```python
from build123d import *

# Parameters (mm, degrees)
PAD_DEPTH            = 70
SKETCH001_W          = 11.887794
SKETCH001_H          = 46.78
POCKET_DEPTH         = 70.001
POCKET001_DEPTH      = 30
SKETCH003_R          = 1.9
POCKET002_DEPTH      = 40.001
SKETCH004_W          = 17
SKETCH004_H          = 23.314381
POCKET003_DEPTH      = 40.001
SKETCH005_W          = 35
SKETCH005_H          = 57.974789
POCKET004_DEPTH      = 26
SKETCH006_W          = 45.255611
SKETCH006_H          = 30.428207
POCKET005_DEPTH      = 28
POCKET005_DEPTH_BACK = -100
SKETCH007_W          = 26.242121
SKETCH007_H          = 29.741062
POCKET006_DEPTH      = 45
SKETCH008_W          = 15.625622
SKETCH008_H          = 14.392597
SKETCH008_W_2        = 24.610352
SKETCH008_H_2        = 31.67345
POCKET007_DEPTH      = 45
SKETCH009_R          = 1.9
POCKET008_DEPTH      = 13
SKETCH010_R          = 1.6
POCKET009_DEPTH      = 5
SKETCH014_W          = 10
SKETCH014_H          = 15
PAD001_DEPTH         = 23
SKETCH015_W          = 11
SKETCH015_H          = 38.184422
SKETCH015_W_2        = 19.881198
SKETCH015_H_2        = 10
PAD002_DEPTH         = 8
SKETCH013_R          = 1.9
POCKET010_DEPTH      = 17
SKETCH011_R          = 1.9
POCKET011_DEPTH      = 15
PAD003_DEPTH         = 5
SKETCH017_R          = 3
POCKET012_DEPTH      = 2


with BuildPart() as part:
    # Sketch → Pad (new body)
    with BuildSketch(Plane.XY):
        Polygon((0, 0), (45, 0), (45, -50), (-28, -50), (-28, 0), align=None)
    extrude(amount=PAD_DEPTH)

    # Sketch001 (on Face7 of Pad) → Pocket (cut, through all)
    with BuildSketch(Plane.XY.offset(70)):
        with Locations((34.056103, -28.39)):
            Rectangle(SKETCH001_W, SKETCH001_H)
    extrude(amount=-POCKET_DEPTH, mode=Mode.SUBTRACT)

    # Sketch002 (on Face5 of Pocket) → Pocket001 (cut)
    with BuildSketch(Plane.XY.offset(70)):
        Polygon((30, -5), (30, -65.096024), (-40.783405, -65.096024), (-40.783405, 12.994774), (20, 12.994774), (20, -5), align=None)
    extrude(amount=-POCKET001_DEPTH, mode=Mode.SUBTRACT)

    # Sketch003 (on Face6 of Pocket001) → Pocket002 (cut, through all)
    with BuildSketch(Plane.XY.offset(40)):
        with Locations((-22, -40)):
            Circle(SKETCH003_R)
        with Locations((22, -40)):
            Circle(SKETCH003_R)
    extrude(amount=-POCKET002_DEPTH, mode=Mode.SUBTRACT)

    # Sketch004 (on Face6 of Pocket002) → Pocket003 (cut, through all)
    with BuildSketch(Plane.XY.offset(40)):
        with Locations((0, -43.65719)):
            Rectangle(SKETCH004_W, SKETCH004_H)
    extrude(amount=-POCKET003_DEPTH, mode=Mode.SUBTRACT)

    # Sketch005 (on Face13 of Pocket003) → Pocket004 (cut)
    with BuildSketch(Plane.XZ.offset(50)):
        with Locations((0, 7.512606)):
            Rectangle(SKETCH005_W, SKETCH005_H)
    extrude(amount=-POCKET004_DEPTH, mode=Mode.SUBTRACT)

    # Sketch006 (on Face11 of Pocket004) → Pocket005 (cut, two sides)
    with BuildSketch(Plane.XZ.offset(24)) as pocket005_sk:
        with Locations((-10.127806, 6.785896)):
            Rectangle(SKETCH006_W, SKETCH006_H)
    extrude(amount=-POCKET005_DEPTH, mode=Mode.SUBTRACT)
    extrude(pocket005_sk.sketch, amount=-POCKET005_DEPTH_BACK, mode=Mode.SUBTRACT)

    # Sketch007 (on Face12 of Pocket005) → Pocket006 (cut)
    with BuildSketch(Plane.XZ.offset(50)):
        with Locations((20.733142, 3.968048)):
            Rectangle(SKETCH007_W, SKETCH007_H)
    extrude(amount=-POCKET006_DEPTH, mode=Mode.SUBTRACT)

    # Sketch008 (on Face14 of Pocket006) → Pocket007 (cut)
    with BuildSketch(Plane.XZ.offset(50)):
        with Locations((42.909006, 69.196298)):
            Rectangle(SKETCH008_W, SKETCH008_H)
        with Locations((46.359665, 3.163275)):
            Rectangle(SKETCH008_W_2, SKETCH008_H_2)
    extrude(amount=-POCKET007_DEPTH, mode=Mode.SUBTRACT)

    # Sketch009 (on Face3 of Pocket007) → Pocket008 (cut)
    with BuildSketch(Plane.YZ.offset(45)):
        with Locations((-44, 55)):
            Circle(SKETCH009_R)
        with Locations((-13, 24)):
            Circle(SKETCH009_R)
        with Locations((-13, 55)):
            Circle(SKETCH009_R)
        with Locations((-44, 24)):
            Circle(SKETCH009_R)
    extrude(amount=-POCKET008_DEPTH, mode=Mode.SUBTRACT)

    # Sketch010 (on Face1 of Pocket008) → Pocket009 (cut)
    with BuildSketch(Plane(origin=(0, 0, 0), x_dir=(-1, 0, 0), z_dir=(0, 1, 0))):
        with Locations((-33, 5)):
            Circle(SKETCH010_R)
        with Locations((-40, 65)):
            Circle(SKETCH010_R)
        with Locations((-26, 65)):
            Circle(SKETCH010_R)
    extrude(amount=-POCKET009_DEPTH, mode=Mode.SUBTRACT)

    # Sketch014 (on Face4 of Pocket009) → Pad001 (join)
    with BuildSketch(Plane.YZ.offset(45)):
        with Locations((-30, 32.5)):
            Rectangle(SKETCH014_W, SKETCH014_H)
    extrude(amount=-PAD001_DEPTH)

    # Sketch015 (on Face29 of Pad001) → Pad002 (join)
    with BuildSketch(Plane(origin=(-28, 0, 0), x_dir=(0, -1, 0), z_dir=(-1, 0, 0))):
        with Locations((13.5, 54.907789)):
            Rectangle(SKETCH015_W, SKETCH015_H)
        with Locations((52.059401, 30)):
            Rectangle(SKETCH015_W_2, SKETCH015_H_2)
    extrude(amount=-PAD002_DEPTH)

    # Sketch013 (on Face19 of Pad002) → Pocket010 (cut)
    with BuildSketch(Plane.XZ.offset(24)):
        with Locations((-7, 27)):
            Circle(SKETCH013_R)
        with Locations((7, 27)):
            Circle(SKETCH013_R)
    extrude(amount=-POCKET010_DEPTH, mode=Mode.SUBTRACT)

    # Sketch011 (on Face29 of Pad002) → Pocket011 (cut)
    with BuildSketch(Plane(origin=(-28, 0, 0), x_dir=(0, -1, 0), z_dir=(-1, 0, 0))):
        with Locations((56.5, 30)):
            Circle(SKETCH011_R)
        with Locations((13, 68.5)):
            Circle(SKETCH011_R)
    extrude(amount=-POCKET011_DEPTH, mode=Mode.SUBTRACT)

    # Sketch016 (on Face1 of Pocket011) → Pad003 (join)
    with BuildSketch(Plane(origin=(0, 0, 0), x_dir=(-1, 0, 0), z_dir=(0, 1, 0))):
        Polygon((-12.5, 0), (5, 22), (-15.71, 22), align=None)
    extrude(amount=-PAD003_DEPTH)

    # Sketch017 (on Face28 of Pad003) → Pocket012 (cut)
    with BuildSketch(Plane.XZ.offset(5)):
        with Locations((26, 65)):
            Circle(SKETCH017_R)
        with Locations((33, 5)):
            Circle(SKETCH017_R)
        with Locations((40, 65)):
            Circle(SKETCH017_R)
    extrude(amount=-POCKET012_DEPTH, mode=Mode.SUBTRACT)


solid = part.part
```
The listing builds one solid part. Answer for the finished solid, in the listing's coordinates (mm). A direction names the side the tool comes from. Coordinates: 2 decimals unless noted, no trailing zeros. Write each loop counter-clockwise with the first axis right and the second up, starting at its lowest first coordinate (ties: lowest second). Pieces come first, ordered by that corner, then holes. Notation, with made-up numbers: (48, 75.25) - (65, 75.25) arc R22 ccw to (65, 98.25) - close; hole circle Ø9 at (86, -8.75). An arc over 180 degrees is marked (long way). Return JSON: item names as keys, results as strings. Group by question number.
1. A cutting plane is placed at C-C, the plane x = 22. Determine the outline of the cut face in (y, z), plus the area to 3 significant figures.
2. Determine the mould class of faces 4 (the flat face through (28.112, -23, 30)), 5 (the flat face through (29, -2, 0)), 6 (the flat face through (40, -28, 41)), 7 (the flat face through (12.5, -15, 20)) for opening direction X: released by +X, released by -X, zero draft, split by the parting line, or undercut.
3. A cutting plane is placed at D-D, the plane x = -22. Determine the outline of the cut face in (y, z), plus the area to 3 significant figures.
4. A cutting plane is placed at A-A, the plane y = -33.5. Determine the outline of the cut face in (x, z), plus the area to 3 significant figures.
5. A cutting plane is placed at B-B, the plane z = 65. Determine the outline of the cut face in (x, y), plus the area to 3 significant figures.
6. Which of the six approach directions +Z, -Z, +X, -X, +Y, -Y give full straight-line access (tool end or side, diameter ignored) to faces 1 (the flat face through (27.3, -3, 63.7)), 2 (the flat face through (0, -31, 36.5)), 3 (the cylindrical face through (42.535, -13.412, 53.145))?
7. Given pin 1 (2 mm diameter, centred on x = 31.5, y = -7.5, fed in from -Z); pin 2 (5 mm diameter, centred on x = 26, z = 65, fed in from -Y); pin 3 (10 mm diameter, centred on y = -45, z = 55, fed in from -X); pin 4 (2.5 mm diameter, centred on x = -23.5, z = 57.5, fed in from -Y), each flat-ended and moving along its own axis, determine where each tip first touches the part or whether it passes through.
8. Straight lines are drawn through the part: L1, parallel to X at y = -37, z = 27; L2, parallel to Z at x = 33, y = -0.8; L3, parallel to X at y = -17, z = 32.5. For each, find the intervals that lie inside material, in ascending order.
Ans:
{
 "1": {"outline": "(-50, 18.84) - (-41.9, 18.84) - (-41.9, 40) - (-50, 40) - close; (-38.1, 18.84) - (-5, 18.84) - (-5, 0) - (0, 0) - (0, 70) - (-5, 70) - (-5, 40) - (-38.1, 40) - close", "area": "1,220 mm²"},
 "2": {"face 4": "undercut", "face 5": "zero draft", "face 6": "undercut", "face 7": "released by -X"},
 "3": {"outline": "(-62, 25) - (-50, 25) - (-50, 22) - (-41.9, 22) - (-41.9, 40) - (-50, 40) - (-50, 35) - (-62, 35) - close; (-38.1, 22) - (0, 22) - (0, 40) - (-8, 40) - (-8, 74) - (-19, 74) - (-19, 40) - (-38.1, 40) - close; hole circle Ø3.8 at (-56.5, 30); hole circle Ø3.8 at (-13, 68.5)", "area": "1,300 mm²"},
 "4": {"outline": "(-28, 22) - (-17.5, 22) - (-17.5, 36.5) - (-8.5, 36.5) - (-8.5, 40) - (-28, 40) - close; (8.5, 36.5) - (17.5, 36.5) - (17.5, 18.84) - (28.11, 18.84) - (28.11, 25) - (40, 25) - (40, 19) - (45, 19) - (45, 62) - (40, 62) - (40, 40) - (8.5, 40) - close", "area": "870 mm²"},
 "5": {"outline": "(-28, -19) - (-20, -19) - (-20, -8) - (-28, -8) - close; (20, -5) - (23, -5) - (23, -3) - (24.4, -3) - (24.4, 0) - (20, 0) - close; (27.6, -3) - (29, -3) - (29, -5) - (37, -5) - (37, -3) - (38.4, -3) - (38.4, 0) - (27.6, 0) - close; (41.6, -3) - (43, -3) - (43, -5) - (45, -5) - (45, 0) - (41.6, 0) - close", "area": "170 mm²"},
 "6": {"face 1": "-Y", "face 2": "-Z, -Y", "face 3": "+X"},
 "7": {"pin 1": "through", "pin 2": "y = -3", "pin 3": "x = 40", "pin 4": "y = -19"},
 "8": {"L1": "-28 to -17.5, 17.5 to 28.11, 40 to 45", "L2": "0 to 3.4, 6.6 to 70", "L3": "-28 to 28.11, 40 to 45"}
}
